For this review, take the finished solid that the model builds, in its own axes (mm). A direction names the side the tool comes from. Coordinates: 2 decimals unless noted, no trailing zeros. Loops run counter-clockwise (first coordinate to the right, second up) from the corner with the lowest first, then second, coordinate; pieces in that order, holes last. Notation, with made-up numbers: M -20,38 L 10,38 A31 cw 10,73 Z; hole C 35.25,4 d4. An arc over 180 degrees is marked long. Put each result on its own line as item: value.
```python
from build123d import *

# Parameters (mm, degrees)
SKETCH1_W           = 31
SKETCH1_H           = 11.43285124
SKETCH1_R           = 1.55
BOSS_EXTRUDE1_DEPTH = 3
SKETCH2_R           = 1.55
CUT_EXTRUDE1_DEPTH  = 31
SKETCH2_3_R         = 2.5
SKETCH2_3_R_2       = 1.55
BOSS_EXTRUDE2_DEPTH = 31
SKETCH3_W           = 25
SKETCH3_H           = 7.5
CUT_EXTRUDE2_DEPTH  = 19.241700852


with BuildPart() as part:
    # Sketch1 → Boss-Extrude1 (new body)
    with BuildSketch(Plane(origin=(0, 0, 0), x_dir=(1, 0, 0), z_dir=(0, 1, 0))):
        Rectangle(SKETCH1_W, SKETCH1_H)
        with Locations(Location((0, -3.21642562, 0), (0, 0, 270))):
            Circle(SKETCH1_R, mode=Mode.SUBTRACT)
        with Locations(Location((5, -3.21642562, 0), (0, 0, 270))):
            Circle(SKETCH1_R, mode=Mode.SUBTRACT)
        with Locations(Location((10, -3.21642562, 0), (0, 0, 270))):
            Circle(SKETCH1_R, mode=Mode.SUBTRACT)
        with Locations(Location((-5, -3.21642562, 0), (0, 0, 270))):
            Circle(SKETCH1_R, mode=Mode.SUBTRACT)
        with Locations(Location((-10, -3.21642562, 0), (0, 0, 270))):
            Circle(SKETCH1_R, mode=Mode.SUBTRACT)
    extrude(amount=BOSS_EXTRUDE1_DEPTH)

    # Sketch2 → Cut-Extrude1 (cut)
    with BuildSketch(Plane.ZY.offset(15.5)):
        with Locations((-5.71642562, 2.5)):
            Circle(SKETCH2_R)
    extrude(amount=-CUT_EXTRUDE1_DEPTH, mode=Mode.SUBTRACT)

    # Sketch2<3> → Boss-Extrude2 (add)
    with BuildSketch(Plane.ZY.offset(15.5)):
        with Locations((-5.71642562, 2.5)):
            Circle(SKETCH2_3_R)
        with Locations((-5.71642562, 2.5)):
            Circle(SKETCH2_3_R_2, mode=Mode.SUBTRACT)
    extrude(amount=-BOSS_EXTRUDE2_DEPTH)

    # Sketch3 → Cut-Extrude2 (cut, through all)
    with BuildSketch(Plane.XZ):
        with Locations((0, -4.46642562)):
            Rectangle(SKETCH3_W, SKETCH3_H)
    extrude(amount=-CUT_EXTRUDE2_DEPTH, mode=Mode.SUBTRACT)


solid = part.part
```
(1) Add section C-C (x = 10). Write out the cut boundary in (y, z), plus the area to 4 significant figures.
Determined:
outline: M 0,-0.72 L 3,-0.72 L 3,1.67 L 0,1.67 Z; M 0,4.77 L 3,4.77 L 3,5.72 L 0,5.72 Z
area: 10.00 mm^2
(2) Wall thickness on line 1 along X through (y, z) = (2.8, 2.25); line 2 along X through (y, z) = (2.35, -4); line 3 along X through (y, z) = (0.9, 2.5): over which ranges is each line inside the solid? List them lowest first. Write a range as [from, to].
Determined:
line 1: x = [-15.5, -11.21], [-8.79, -6.21], [-3.79, -1.21], [1.21, 3.79], [6.21, 8.79], [11.21, 15.5]
line 2: x = [-15.5, -12.5], [12.5, 15.5]
line 3: x = [-15.5, -11.37], [-8.63, -6.37], [-3.63, -1.37], [1.37, 3.63], [6.37, 8.63], [11.37, 15.5]
(3) Add section B-B (z = -1.75). Write out the cut boundary in (x, y), plus the area to 3 significant figures.
Determined:
outline: M -15.5,0 L -12.5,0 L -12.5,3 L -15.5,3 Z; M 12.5,0 L 15.5,0 L 15.5,3 L 12.5,3 Z
area: 18.0 mm^2
(4) Add section D-D (z = 3.75). Write out the cut boundary in (x, y).
Determined:
outline: M -15.5,0 L -11.46,0 L -11.46,3 L -15.5,3 Z; M -8.54,0 L -6.46,0 L -6.46,3 L -8.54,3 Z; M -3.54,0 L -1.46,0 L -1.46,3 L -3.54,3 Z; M 1.46,0 L 3.54,0 L 3.54,3 L 1.46,3 Z; M 6.46,0 L 8.54,0 L 8.54,3 L 6.46,3 Z; M 11.46,0 L 15.5,0 L 15.5,3 L 11.46,3 Z
(5) Tool access review of faces 5 (the cylindrical face through (-10.59, 1.48, 4.65)), 6 (the flat face through (-12.5, 2, -4)): name each direction out of +Z, -Z, +X, -X, +Y, -Y from which nothing blocks a thin tool from reaching the whole face with its end or side.
Determined:
face 5: +Y, -Y
face 6: -Z, +Y, -Y
(6) For pin 1 (8 mm diameter, centred on x = 7.5, z = 3.5, fed in from +Y), flat-tipped, find the tip position at first contact; note if it passes through.
Determined:
pin 1: stops at y = 3
(7) Draft analysis for pull direction X (two halves, no side actions). For faces 1 (the cylindrical face through (-0.59, 1.48, 4.65)), 2 (the flat face through (15.5, 2, -1)), 3 (the flat face through (0, 3, 1)), 4 (the flat face through (0, 1, -0.716)), state which applies: +X half, -X half, draft (parallel to the pull), parting line (faces both ways), or undercut.
Determined:
face 1: undercut
face 2: +X half
face 3: draft
face 4: undercut
(8) Add section A-A (y = 2.5). Write out the cut boundary in (x, z).
Determined:
outline: M -15.5,-8.22 L -12.5,-8.22 L -12.5,-7.27 L -15.5,-7.27 Z; M -15.5,-4.17 L -12.5,-4.17 L -12.5,-0.72 L 12.5,-0.72 L 12.5,-4.17 L 15.5,-4.17 L 15.5,5.72 L -15.5,5.72 Z; M 12.5,-8.22 L 15.5,-8.22 L 15.5,-7.27 L 12.5,-7.27 Z; hole C -10,3.22 d3.1; hole C -5,3.22 d3.1; hole C 0,3.22 d3.1; hole C 5,3.22 d3.1; hole C 10,3.22 d3.1
